```python
from build123d import *

# Parameters (mm, degrees)
SKETCH008_W      = 57.25
SKETCH008_H      = 78
PAD004_DEPTH     = 2
SKETCH009_W      = 61.25
SKETCH009_H      = 82
PAD005_DEPTH     = 2
PAD006_DEPTH     = 4
POCKET004_DEPTH  = 20
HOLE_D           = 3.4
HOLE_DEPTH       = 25
HOLE_CSINK_D     = 6.1
HOLE_CSINK_ANGLE = 90
FILLET003_R      = 3
FILLET004_R      = 4
FILLET005_R      = 1.5
FILLET006_R      = 6


with BuildPart() as part:
    # Sketch008 → Pad004 (new body)
    with BuildSketch(Plane.XY):
        with Locations((-8.875, 0)):
            Rectangle(SKETCH008_W, SKETCH008_H)
        with BuildLine():
            ThreePointArc((-13.5, 30.25), (-10, 26.75), (-6.5, 30.25))
            Line((-6.5, 30.25), (-6.5, 38))
            Line((-6.5, 38), (18.75, 38))
            Line((18.75, 38), (18.75, 11.75))
            Line((15, 11.75), (18.75, 11.75))
            ThreePointArc((15, 11.75), (11.5, 8.25), (15, 4.75))
            Line((15, 4.75), (18.75, 4.75))
            Line((18.75, 4.75), (18.75, -38))
            Line((18.75, -38), (-28.5, -38))
            Line((-28.5, -33.75), (-28.5, -38))
            ThreePointArc((-28.5, -33.75), (-29.525126, -31.275126), (-32, -30.25))
            Line((-32, -30.25), (-36.5, -30.25))
            Line((-36.5, -30.25), (-36.5, 38))
            Line((-36.5, 38), (-13.5, 38))
            Line((-13.5, 30.25), (-13.5, 38))
        make_face(mode=Mode.SUBTRACT)
    extrude(amount=-PAD004_DEPTH)

    # Sketch009 → Pad005 (join)
    with BuildSketch(Plane.XY):
        with Locations((-8.625, 0)):
            Rectangle(SKETCH009_W, SKETCH009_H)
    extrude(amount=PAD005_DEPTH)

    # Sketch010 (on DatumPlane) → Pad006 (join)
    with BuildSketch(Plane.XY.offset(2)):
        Polygon((-13.5, -33), (-9, -33), (-9, -41), (9, -41), (9, -33), (13.5, -33), (13.5, -9), (9, -9), (9, 26), (-9, 26), (-9, -9), (-13.5, -9), align=None)
    extrude(amount=PAD006_DEPTH)

    # Sketch011 (on DatumPlane) → Pocket004 (cut)
    with BuildSketch(Plane.XZ.offset(31)):
        Polygon((-17.5, 7), (-17.5, 0), (17.5, 0), (17.5, 7), (13.5, 7), (13.5, 2), (-13.5, 2), (-13.5, 7), align=None)
    extrude(amount=-POCKET004_DEPTH, mode=Mode.SUBTRACT)

    # Hole
    with Locations(Plane.XY.offset(2)):
        with Locations((-32, -33.75), (-10, 30.25), (15, 8.25)):
            CounterSinkHole(HOLE_D / 2, HOLE_CSINK_D / 2, depth=HOLE_DEPTH, counter_sink_angle=HOLE_CSINK_ANGLE)

    # Fillet003
    fillet003_edges = [part.edges().sort_by_distance(p)[0] for p in [
        (18.75, 4.75, -1),
        (18.75, 11.75, -1),
        (-6.5, 38, -1),
        (-13.5, 38, -1),
        (-36.5, -30.25, -1),
        (-28.5, -38, -1),
        (-36.5, 38, -1),
        (18.75, -38, -1),
        (18.75, 38, -1),
    ]]
    fillet(fillet003_edges, radius=FILLET003_R)

    # Fillet004
    fillet004_edges = [part.edges().sort_by_distance(p)[0] for p in [
        (19.75, -39, -1),
        (-37.5, -39, -1),
        (19.75, 39, -1),
        (-37.5, 39, -1),
    ]]
    fillet(fillet004_edges, radius=FILLET004_R)

    # Fillet005
    fillet005_edges = [part.edges().sort_by_distance(p)[0] for p in [
        (9, -41, 4),
        (-9, -41, 4),
        (13.5, -9, 4),
        (9, 26, 4),
        (-9, 26, 4),
        (-13.5, -9, 4),
        (-13.5, -33, 4),
        (13.5, -33, 4),
    ]]
    fillet(fillet005_edges, radius=FILLET005_R)

    # Fillet006
    fillet006_edges = [part.edges().sort_by_distance(p)[0] for p in [
        (-39.25, -41, 1),
        (22, -41, 1),
        (22, 41, 1),
        (-39.25, 41, 1),
    ]]
    fillet(fillet006_edges, radius=FILLET006_R)


solid = part.part
```
The listing builds one solid part. Answer for the finished solid, in the listing's coordinates (mm). A direction names the side the tool comes from. Round coordinates to 2 decimals unless told otherwise and drop trailing zeros. Loops run counter-clockwise (first coordinate to the right, second up) from the corner with the lowest first, then second, coordinate; pieces in that order, holes last.
Q1. Section C-C, the plane x = -21 is taken. Determine the outline of the cut face in (y, z).
Q2. Find the intervals of material crossed by line 1 (Y direction, x = -10, z = -1.3); line 2 (X direction, y = 8.25, z = -1.4); line 3 (X direction, y = 30.25, z = -0.7), in increasing order.
Q3. Section D-D, the plane y = 13 is taken. Determine the outline of the cut face in (x, z).
Q4. Which of the six approach directions +Z, -Z, +X, -X, +Y, -Y give full straight-line access (tool end or side, diameter ignored) to faces 4 (the face through (-36.359, -37.797, -1.014)), 5 (the face through (9, 8, 4)), 6 (the face through (0, -31, 1))?
Q5. Given pin 1 Ø2 at (x, z) = (-27, -0.5) entering from -Y; pin 2 Ø4 at (x, y) = (-8.5, 29) entering from +Z; pin 3 Ø2 at (y, z) = (19.5, 4) entering from +X; pin 4 Ø0.6 at (x, z) = (4, -0.5) entering from +Y, each flat-ended and moving along its own axis, determine where each tip first touches the part or whether it passes through.
Q6. Section A-A, the plane x = -10 is taken. Determine the outline of the cut face in (y, z).
Q7. For a pull along Y with two mould halves and no side action, classify faces 1 (the face through (10, -33, 4)), 2 (the face through (-27.6, -37.14, -1.01)), 3 (the face through (-13.5, -21, 4)) as released by +Y, released by -Y, zero draft, split by the parting line, or undercut.
Q8. Section B-B, the plane z = 4.5 is taken. Determine the outline of the cut face in (x, y), then the cut area to 3 significant figures.
Completed:
1. outline: (-41, 0) - (-39, 0) - (-39, -2) - (-38, -2) - (-38, 0) - (38, 0) - (38, -2) - (39, -2) - (39, 0) - (41, 0) - (41, 2) - (-41, 2) - close
2. line 1: y = -39 to -38, 26.75 to 28.55, 31.95 to 39
2. line 2: x = -37.5 to -36.5, 11.5 to 13.3, 16.7 to 19.75
2. line 3: x = -37.5 to -36.5, -13.5 to -11.7, -8.3 to -6.5, 18.75 to 19.75
3. outline: (-39.25, 0) - (-37.5, 0) - (-37.5, -2) - (-36.5, -2) - (-36.5, 0) - (18.19, 0) - (18.19, -2) - (19.75, -2) - (19.75, 0) - (22, 0) - (22, 2) - (9, 2) - (9, 6) - (-9, 6) - (-9, 2) - (-39.25, 2) - close
4. face 4: -Z, -X, -Y
4. face 5: +Z, +X, +Y
4. face 6: -Z
5. pin 1: stops at y = -41
5. pin 2: stops at z = 2
5. pin 3: stops at x = 9
5. pin 4: stops at y = 39
6. outline: (-41, 0) - (-39, 0) - (-39, -2) - (-38, -2) - (-38, 0) - (-31, 0) - (-31, 2) - (-11, 2) - (-11, 0) - (26.75, 0) - (26.75, -2) - (28.55, -2) - (28.55, 0.65) - (27.2, 2) - (-9, 2) - (-9, 6) - (-33, 6) - (-33, 2) - (-41, 2) - close; (31.95, -2) - (39, -2) - (39, 0) - (41, 0) - (41, 2) - (33.3, 2) - (31.95, 0.65) - close
7. face 1: released by -Y
7. face 2: undercut
7. face 3: zero draft
8. outline: (-13.5, -31.5) arc R1.5 ccw to (-12, -33) - (-9, -33) - (-9, -39.5) arc R1.5 ccw to (-7.5, -41) - (7.5, -41) arc R1.5 ccw to (9, -39.5) - (9, -33) - (12, -33) arc R1.5 ccw to (13.5, -31.5) - (13.5, -10.5) arc R1.5 ccw to (12, -9) - (9, -9) - (9, 24.5) arc R1.5 ccw to (7.5, 26) - (-7.5, 26) arc R1.5 ccw to (-9, 24.5) - (-9, -9) - (-12, -9) arc R1.5 ccw to (-13.5, -10.5) - close
8. area: 1,420 mm2
